from build123d import *

# Parameters (mm, degrees)
BOSS_EXTRUDE1_DEPTH = 107.95
CUT_EXTRUDE1_REACH  = 114.802
SKETCH2_R           = 3.175
CUT_EXTRUDE2_REACH  = 115.77
SKETCH3_R           = 3.175


with BuildPart() as part:
    # Sketch1 → Boss-Extrude1 (new body)
    with BuildSketch(Plane(origin=(0, 0, 0), x_dir=(0, 0, -1), z_dir=(1, 0, 0))):
        Polygon((0, 0), (0, -25.4), (25.4, -25.4), (25.4, -20.6375), (4.7625, -20.6375), (4.7625, 0), align=None)
    extrude(amount=BOSS_EXTRUDE1_DEPTH)

    # Sketch2 → Cut-Extrude1 (cut, up to next)
    with BuildSketch(Plane(origin=(0, -20.6375, 0), x_dir=(1, 0, 0), z_dir=(0, 1, 0)), mode=Mode.PRIVATE) as cut_extrude1_sk1:
        with Locations(Location((9.525, 11.1125, 0), (0, 0, 270))):
            Circle(SKETCH2_R)
    cut_extrude1_tool1 = extrude(cut_extrude1_sk1.sketch, amount=-CUT_EXTRUDE1_REACH, mode=Mode.PRIVATE) & part.part
    # Sketch2 → Cut-Extrude1 (cut, up to next)
    with BuildSketch(Plane(origin=(0, -20.6375, 0), x_dir=(1, 0, 0), z_dir=(0, 1, 0)), mode=Mode.PRIVATE) as cut_extrude1_sk2:
        with Locations(Location((19.05, 17.4625, 0), (0, 0, 270))):
            Circle(SKETCH2_R)
    cut_extrude1_tool2 = extrude(cut_extrude1_sk2.sketch, amount=-CUT_EXTRUDE1_REACH, mode=Mode.PRIVATE) & part.part
    add(cut_extrude1_tool1.solids().sort_by_distance((9.525, -20.6375, -11.1125))[0], mode=Mode.SUBTRACT)
    add(cut_extrude1_tool2.solids().sort_by_distance((19.05, -20.6375, -17.4625))[0], mode=Mode.SUBTRACT)

    # Sketch3 → Cut-Extrude2 (cut, up to next)
    with BuildSketch(Plane.XZ.offset(25.4), mode=Mode.PRIVATE) as cut_extrude2_sk1:
        with Locations(Location((76.332177029, -13.470384182, 0), (0, 0, 270))):
            Circle(SKETCH3_R)
    cut_extrude2_tool1 = extrude(cut_extrude2_sk1.sketch, amount=-CUT_EXTRUDE2_REACH, mode=Mode.PRIVATE) & part.part
    add(cut_extrude2_tool1.solids().sort_by_distance((76.332177, -25.4, -13.470384))[0], mode=Mode.SUBTRACT)


solid = part.part
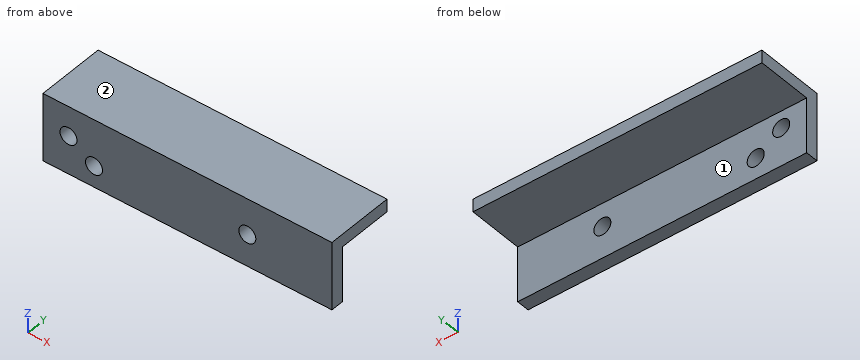
CAD build for the part. Positions are in the model's coordinates, mm. Face numbers are marked on the shaded views. A direction names the side the tool comes from. Round coordinates to 2 decimals unless told otherwise and drop trailing zeros. Loops run counter-clockwise (first coordinate to the right, second up) from the corner with the lowest first, then second, coordinate; pieces in that order, holes last.
(1) Cut at B-B (y = -22). State how many separate pieces and enclosed holes the cut face has, plus the area to 3 significant figures.
(2) Wall check: line 1 along Y through (x, z) = (48, -5.75); line 2 along Z through (x, y) = (92, -7.75); line 3 along X through (y, z) = (-24, -10.75). Give the ranges that are in metal, low to high.
(3) Cut at C-C (z = -21.75). Give the cut face in (x, y).
(4) Cut at D-D (x = 96.5). Give the cut face in (y, z), plus the area to 3 significant figures.
(5) Which spindle directions (+Z, -Z, +X, -X, +Y, -Y) get a long thin tool onto all of the face, cutting with end or side? Do the marked faces 1 and 2. Say none if no direction does.
(6) Cut at A-A (x = 19.05). Give the cut face in (y, z).
(7) Drop flat-ended pins along their axis: pin 1 (10 mm diameter, centred on x = 76.33, z = -13.47, fed in from -Y); pin 2 (10.5 mm diameter, centred on x = 39.5, z = -12, fed in from +Y). Give the stop position or say it passes through.
Findings below:
1. separate pieces: 1
1. enclosed holes: 3
1. area: 2,650 mm2
2. line 1: y = -25.4 to -20.64
2. line 2: z = -4.76 to 0
2. line 3: x = 0 to 6.37, 12.68 to 74.7, 77.97 to 107.95
3. outline: (0, -25.4) - (107.95, -25.4) - (107.95, -20.64) - (0, -20.64) - close
4. outline: (-25.4, -25.4) - (-20.64, -25.4) - (-20.64, -4.76) - (0, -4.76) - (0, 0) - (-25.4, 0) - close
4. area: 219 mm2
5. face 1: -Z, +X, -X, +Y
5. face 2: +Z, +X, -X, +Y, -Y
6. outline: (-25.4, -25.4) - (-20.64, -25.4) - (-20.64, -20.64) - (-25.4, -20.64) - close; (-25.4, -14.29) - (-20.64, -14.29) - (-20.64, -4.76) - (0, -4.76) - (0, 0) - (-25.4, 0) - close
7. pin 1: stops at y = -25.4
7. pin 2: stops at y = -20.64
